Work out the finished part from the listing and answer in its coordinate system (mm). Face numbers are marked on the shaded views. A direction names the side the tool comes from. Give positions to 0.01 mm unless a question says otherwise; leave off trailing zeros. Loops run counter-clockwise (first coordinate to the right, second up) from the corner with the lowest first, then second, coordinate; pieces in that order, holes last. Notation, with made-up numbers: (-18, 74) - (32, 74) arc R20 ccw to (32, 101) - close; hole circle Ø4 at (2, 49). An arc over 180 degrees is marked (long way). Use one line per item in the form item = value. Start each with the question number.
from build123d import *

# Parameters (mm, degrees)
SKETCH1_R           = 10.795
BOSS_EXTRUDE1_DEPTH = 12.7
SKETCH2_R           = 4.7625
BOSS_EXTRUDE2_DEPTH = 17.145
SKETCH3_OUTSIDE_W   = 32.13
SKETCH3_OUTSIDE_H   = 32.13
SKETCH3_OUTSIDE_R   = 3.175
CUT_EXTRUDE1_DEPTH  = 9.525


with BuildPart() as part:
    # Sketch1 → Boss-Extrude1 (new body)
    with BuildSketch(Plane(origin=(0, 0, 0), x_dir=(1, 0, 0), z_dir=(0, 1, 0))):
        Circle(SKETCH1_R)
    extrude(amount=BOSS_EXTRUDE1_DEPTH)

    # Sketch2 → Boss-Extrude2 (add)
    with BuildSketch(Plane.XZ):
        Circle(SKETCH2_R)
    extrude(amount=BOSS_EXTRUDE2_DEPTH)

    # Sketch3 outside → Cut-Extrude1 (cut)
    with BuildSketch(Plane.XZ.offset(17.145)):
        Rectangle(SKETCH3_OUTSIDE_W, SKETCH3_OUTSIDE_H)
        Circle(SKETCH3_OUTSIDE_R, mode=Mode.SUBTRACT)
    extrude(amount=-CUT_EXTRUDE1_DEPTH, mode=Mode.SUBTRACT)


solid = part.part
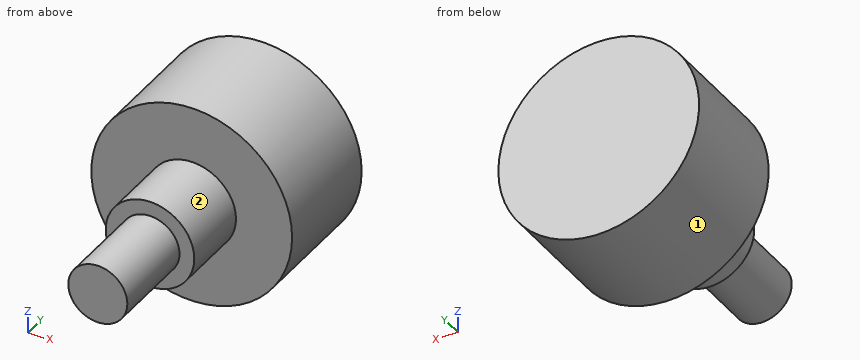
1) Flat-ended cylindrical pins translate along their axes: pin 1 Ø1.5 at (x, y) = (-5, 0) entering from +Z; pin 2 Ø2 at (x, y) = (-3, 5) entering from +Z; pin 3 Ø8 at (x, z) = (-6.5, 8) entering from -Y. Find the tip coordinate at first contact, or state that the pin passes through.
2) A cutting plane is placed at D-D (z = -4.25). Give the vertices of the cut face in (x, y), plus the area to 3 significant figures.
3) A tool of negligible diameter and unlimited length cuts with its end or side. For the marked faces 1 and 2, from which of +Z, -Z, +X, -X, +Y, -Y can it reach the whole face along a straight path? Write none if from no direction.
4) A cutting plane is placed at B-B (x = 0). Give the vertices of the cut face in (y, z) (1 decimal).
5) A cutting plane is placed at C-C (y = 0.5). Give the vertices of the cut face in (x, z) (3 decimals), plus the area to 3 significant figures.
6) A cutting plane is placed at A-A (z = 0). Give the vertices of the cut face in (x, y) (1 decimal).
7) Find the intervals of material crossed by probe 1 along Y at (x, z) = (5.5, -4); probe 2 along Y at (x, z) = (-3.25, 1.25); probe 3 along X at (y, z) = (7.25, 10), in increasing order.
Answer sheet:
q1.pin_1 = 9.92
q1.pin_2 = 10.61
q1.pin_3 = 0
q2.outline = (-9.92, 0) - (-2.15, 0) - (-2.15, -7.62) - (2.15, -7.62) - (2.15, 0) - (9.92, 0) - (9.92, 12.7) - (-9.92, 12.7) - close
q2.area = 285 mm²
q3.face_1 = +Y, -Y
q3.face_2 = -Y
q4.outline = (-17.1, -3.2) - (-7.6, -3.2) - (-7.6, -4.8) - (0, -4.8) - (0, -10.8) - (12.7, -10.8) - (12.7, 10.8) - (0, 10.8) - (0, 4.8) - (-7.6, 4.8) - (-7.6, 3.2) - (-17.1, 3.2) - close
q5.outline = circle Ø21.59 at (0, 0)
q5.area = 366 mm²
q6.outline = (-10.8, 0) - (-4.8, 0) - (-4.8, -7.6) - (-3.2, -7.6) - (-3.2, -17.1) - (3.2, -17.1) - (3.2, -7.6) - (4.8, -7.6) - (4.8, 0) - (10.8, 0) - (10.8, 12.7) - (-10.8, 12.7) - close
q7.probe_1 = 0 to 12.7
q7.probe_2 = -7.62 to 12.7
q7.probe_3 = -4.07 to 4.07
